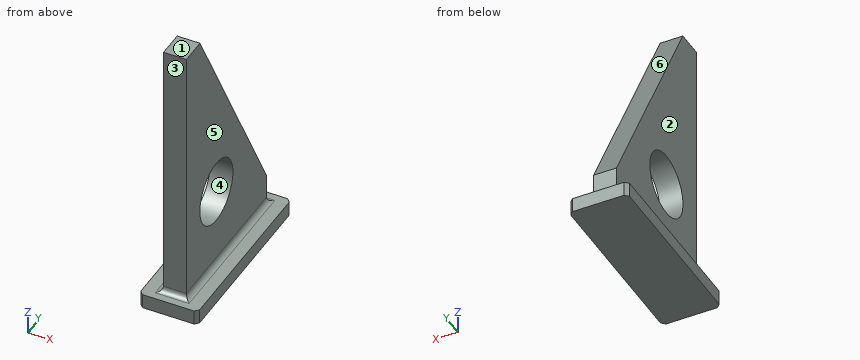
```python
from build123d import *

# Parameters (mm, degrees)
EXTRUDE8_DEPTH  = 15.748
SKETCH8_R       = 22.225
EXTRUDE10_DEPTH = 215.740536803
SKETCH9_W       = 40.631586246
SKETCH9_H       = 125.535865236
EXTRUDE11_DEPTH = 10.16
CHAMFER1_SIZE   = 2.54
FILLET2_R       = 3.81


with BuildPart() as part:
    # Sketch7 → Extrude8 (new body)
    with BuildSketch(Plane(origin=(0, 0, 0), x_dir=(0, 0, -1), z_dir=(1, 0, 0))):
        Polygon((-21.030060514, 104.974134166), (-186.670645251, 15.683506456), (-186.670645251, -2.54), (2.54, -2.54), (2.54, 104.974134166), align=None)
    extrude(amount=EXTRUDE8_DEPTH)

    # Sketch8 → Extrude10 (cut, through all)
    with BuildSketch(Plane(origin=(0, 0, 0), x_dir=(0, 0, -1), z_dir=(1, 0, 0))):
        with Locations(Location((-55.180628977, 37.768492455, 0), (0, 0, 180))):
            Circle(SKETCH8_R)
    extrude(amount=EXTRUDE10_DEPTH, mode=Mode.SUBTRACT)

    # Sketch9 → Extrude11 (add)
    with BuildSketch(Plane.XY):
        with Locations((7.874, 51.217067083)):
            Rectangle(SKETCH9_W, SKETCH9_H)
    extrude(amount=-EXTRUDE11_DEPTH)

    # Chamfer1
    chamfer1_edges = [part.edges().sort_by_distance(p)[0] for p in [
        (28.189793123, 113.984999701, -5.08),
        (28.189793123, -11.550865535, -5.08),
        (-12.441793123, -11.550865535, -5.08),
        (-12.441793123, 113.984999701, -5.08),
    ]]
    chamfer(chamfer1_edges, length=CHAMFER1_SIZE)

    # Fillet2
    fillet2_edges = [part.edges().sort_by_distance(p)[0] for p in [
        (7.874, -2.54, 0),
        (15.748, 51.217067083, 0),
        (7.874, 104.974134166, 0),
        (0, 51.217067083, 0),
    ]]
    fillet(fillet2_edges, radius=FILLET2_R)


solid = part.part
```
CAD build for the part. Positions are in the model's coordinates, mm. Face numbers are marked on the shaded views. A direction names the side the tool comes from. Coordinates: 2 decimals unless noted, no trailing zeros. Order: outer loops, then holes, each group sorted by start corner. A loop starts at its lowest first (then second) coordinate and runs counter-clockwise, first axis right, second up. Notation, with made-up numbers: (0.25, 54.5) -> (54.25, 54.5) arc R30 ccw to (54.25, 83.5) -> close; hole circle Ø2 at (39.25, 79.25). An arc over 180 degrees is marked (long way). Use one line per item in the form item = value. Start each with the question number.
1) Band-saw the part on A-A on y = 7. Give the cut face in (x, z).
2) Drill centre lines: L1, parallel to X at y = 27.5, z = 103; L2, parallel to Z at x = 19.5, y = 107.5; L3, parallel to Y at x = 3, z = 37. Where is each one in solid material? Low to high. Write a range as [from, to].
3) Tool access for the marked faces 1, 2 and 3: list every direction of +Z, -Z, +X, -X, +Y, -Y with a clear straight run to the whole face (end or side of a thin tool).
4) Band-saw the part on C-C on z = 151. Give the cut face in (x, y).
5) Band-saw the part on D-D on x = 22. Give the cut face in (y, z) (3 decimals), then the cut area to 3 significant figures.
6) Pull direction Y, two halves, no side cores. Call the marked faces 4, 5 and 6: +Y half, -Y half, draft (parallel to the pull), parting line (faces both ways), or undercut.
7) Drop flat-ended pins along their axis: pin 1 (8 mm diameter, centred on y = 18.5, z = 15.5, fed in from +X); pin 2 (10 mm diameter, centred on x = 6, y = 55, fed in from +Z); pin 3 (8 mm diameter, centred on x = -5.5, y = 93, fed in from +Z). Give the stop position or say it passes through.
Entries:
q1.outline = (-12.44, -10.16) -> (28.19, -10.16) -> (28.19, 0) -> (19.56, 0) arc R3.81 cw to (15.75, 3.81) -> (15.75, 186.67) -> (0, 186.67) -> (0, 3.81) arc R3.81 cw to (-3.81, 0) -> (-12.44, 0) -> close
q2.L1 = [0, 15.75]
q2.L2 = [-10.16, 0]
q2.L3 = [-2.54, 24.99], [50.55, 96.37]
q3.face_1 = +Z, +X, -X, +Y, -Y
q3.face_2 = +Z, -X, +Y, -Y
q3.face_3 = +Z, +X, -X, -Y
q4.outline = (0, -2.54) -> (15.75, -2.54) -> (15.75, 34.91) -> (0, 34.91) -> close
q5.outline = (-11.551, -10.16) -> (113.985, -10.16) -> (113.985, 0) -> (-11.551, 0) -> close
q5.area = 1,280 mm2
q6.face_4 = undercut
q6.face_5 = draft
q6.face_6 = +Y half
q7.pin_1 = 15.75
q7.pin_2 = 123.01
q7.pin_3 = 0.78
